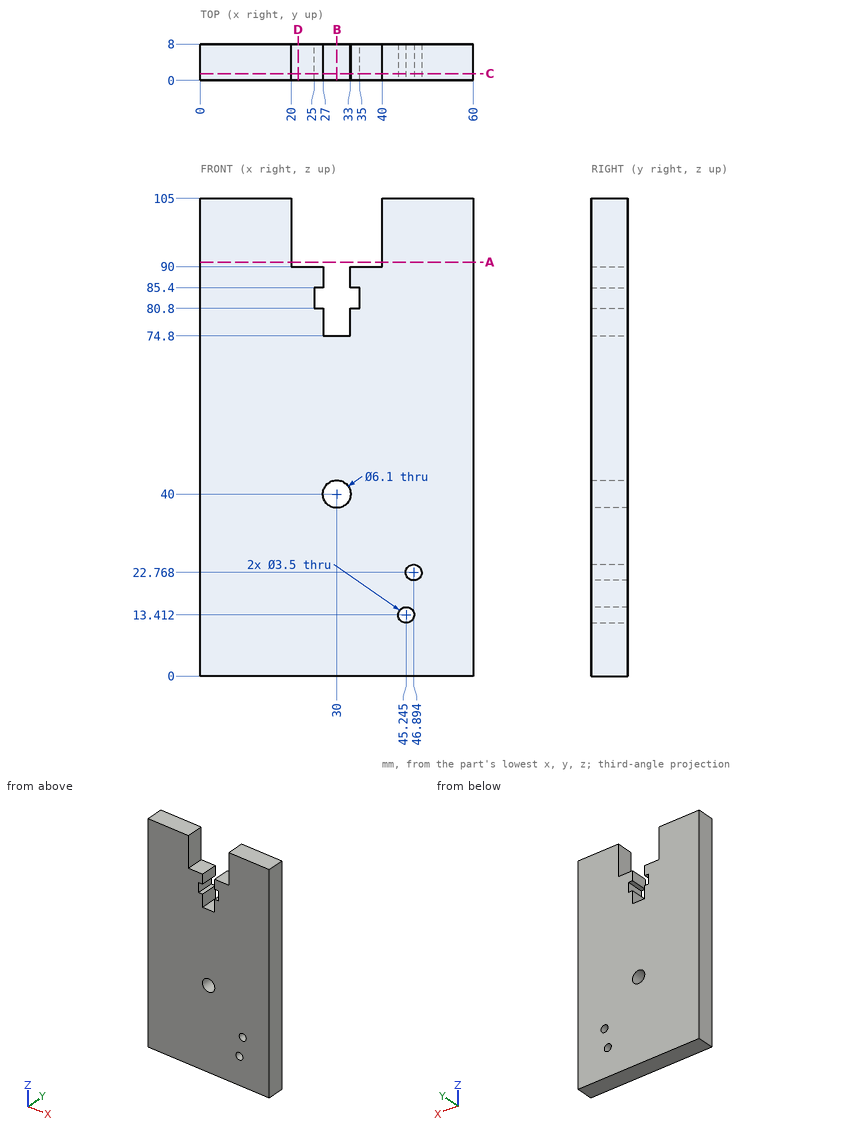
Check sheet for the drawn part. Datum: minimum x, y, z corner. Units: mm. Coordinates: 2 decimals unless noted, no trailing zeros. Write each loop counter-clockwise with the first axis right and the second up, starting at its lowest first coordinate (ties: lowest second). Pieces come first, ordered by that corner, then holes. Notation, with made-up numbers: (39, -14) - (88, -14) arc R27 ccw to (88, 15) - close; hole circle Ø5 at (49.5, 69). An arc over 180 degrees is marked (long way). Answer as a JSON object with one key per item and string values.
(1) Cross-section at B-B on x = 30. Record the cut outline in (y, z).
Report:
{"outline": "(0, 0) - (8, 0) - (8, 36.95) - (0, 36.95) - close; (0, 43.05) - (8, 43.05) - (8, 74.8) - (0, 74.8) - close"}
(2) Cross-section at C-C on y = 1.5. Give the number of separate pieces and of enclosed holes in the cut face, plus the area to 3 significant figures.
Report:
{"separate pieces": "1", "enclosed holes": "3", "area": "5,840 mm^2"}
(3) Thickness scan on line 1 along Z through (x, y) = (25.5, 5); line 2 along X through (y, z) = (7.75, 87.5); line 3 along Z through (x, y) = (45.5, 6) (1 decimal). Record the ranges inside material, lowest first.
Report:
{"line 1": "0 to 80.8, 85.4 to 90", "line 2": "0 to 27, 33 to 60", "line 3": "0 to 11.7, 15.1 to 21.7, 23.8 to 105"}
(4) Cross-section at A-A on z = 91. Record the cut outline in (x, y), plus the area to 3 significant figures.
Report:
{"outline": "(0, 0) - (20, 0) - (20, 8) - (0, 8) - close; (40, 0) - (60, 0) - (60, 8) - (40, 8) - close", "area": "320 mm^2"}
(5) Cross-section at D-D on x = 21.5. Record the cut outline in (y, z), plus the area to 3 significant figures.
Report:
{"outline": "(0, 0) - (8, 0) - (8, 90) - (0, 90) - close", "area": "720 mm^2"}
(6) Gauge pin test, flat ends, axial feed: pin 1 Ø2.5 at (y, z) = (5.5, 96.5) entering from -X; pin 2 Ø1 at (x, y) = (34, 3.5) entering from +Z. Record the tip position at first contact, or that the pin passes through.
Report:
{"pin 1": "x = 0", "pin 2": "z = 90"}
